from build123d import *

# Parameters (mm, degrees)
SKETCH1_W               = 19.5
SKETCH1_H               = 7
BOSS_EXTRUDE1_DEPTH     = 3
CUT_EXTRUDE1_DEPTH      = 7
CUT_EXTRUDE2_DEPTH      = 21.934421415
CUT_EXTRUDE2_DEPTH_BACK = 21.934421415
SKETCH4_R               = 1.8
CUT_EXTRUDE3_DEPTH      = 0.8


with BuildPart() as part:
    # Sketch1 → Boss-Extrude1 (new body)
    with BuildSketch(Plane(origin=(0, 0, 0), x_dir=(1, 0, 0), z_dir=(0, 1, 0))):
        with Locations((9.75, 3.5)):
            Rectangle(SKETCH1_W, SKETCH1_H)
    extrude(amount=BOSS_EXTRUDE1_DEPTH)

    # Sketch2 → Cut-Extrude1 (cut)
    with BuildSketch(Plane.XY):
        Polygon((0, 0), (0.7, 3), (0, 3), align=None)
        Polygon((19.5, 0), (18.8, 3), (19.5, 3), align=None)
    extrude(amount=-CUT_EXTRUDE1_DEPTH, mode=Mode.SUBTRACT)

    # Sketch3 → Cut-Extrude2 (cut, two sides: drawn at the far end of the back side and taken through both)
    with BuildSketch(Plane(origin=(0, 0, 0), x_dir=(0, 0, -1), z_dir=(1, 0, 0)).offset(-CUT_EXTRUDE2_DEPTH_BACK)):
        Polygon((0, 0), (0.7, 3), (0, 3), align=None)
        Polygon((7, 3), (6.3, 3), (7, 0), align=None)
    extrude(amount=CUT_EXTRUDE2_DEPTH + CUT_EXTRUDE2_DEPTH_BACK, mode=Mode.SUBTRACT)

    # Sketch4 → Cut-Extrude3 (cut)
    with BuildSketch(Plane.XZ):
        with Locations(Location((9.75, -3.5, 0), (0, 0, 270))):
            Circle(SKETCH4_R)
    extrude(amount=-CUT_EXTRUDE3_DEPTH, mode=Mode.SUBTRACT)


solid = part.part
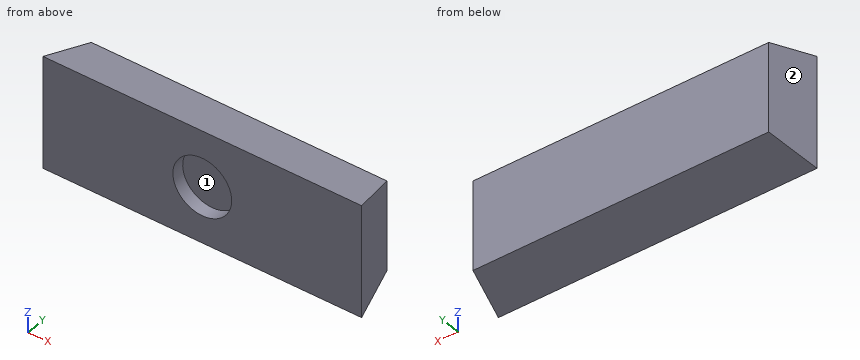
Verification items for the finished model (mm, model axes). Face numbers are marked on the shaded views. Give positions to 0.01 mm unless a question says otherwise; leave off trailing zeros. Order: outer loops, then holes, each group sorted by start corner. A loop starts at its lowest first (then second) coordinate and runs counter-clockwise, first axis right, second up. Notation, with made-up numbers: (89, -29) -> (118, -29) arc R19 ccw to (118, -24) -> close; hole circle Ø2 at (19, 13.25). An arc over 180 degrees is marked (long way). Answer as CSV lines item,"result".
Q1. Scan lines: probe 1 along Y at (x, z) = (9.5, -4.25); probe 2 along X at (y, z) = (0.4, -3.5); probe 3 along Z at (x, y) = (8.5, 0.3). Record each from-to range of solid material in increasing order.
Solutions:
probe 1,"y = 0.8 to 3"
probe 2,"x = 0.09 to 7.95, 11.55 to 19.41"
probe 3,"z = -6.93 to -4.8, -2.2 to -0.07"
Q2. Depth check by flat-ended pin: pin 1 (1.5 mm diameter, centred on y = 1, z = -2.5, fed in from -X). Enter the tip coordinate at first touch or a pass-through.
Solutions:
pin 1,"stops at x = 0.06"
Q3. Sectioned sample at B-B on z = -3.5. Record the cut outline in (x, y), plus the area to 3 significant figures.
Solutions:
outline,"(0, 0) -> (7.95, 0) -> (7.95, 0.8) -> (11.55, 0.8) -> (11.55, 0) -> (19.5, 0) -> (18.8, 3) -> (0.7, 3) -> close"
area,"53.5 mm²"
Q4. Release check for a two-part mould opening along Y. For the marked faces 1 and 2 record: +Y half, -Y half, draft (parallel to the pull), parting line (faces both ways), or undercut.
Solutions:
face 1,"-Y half"
face 2,"+Y half"
Q5. Sectioned sample at D-D on x = 14.5. Record the cut outline in (y, z).
Solutions:
outline,"(0, -7) -> (3, -6.3) -> (3, -0.7) -> (0, 0) -> close"
Q6. Sectioned sample at A-A on x = 9.75. Record the cut outline in (y, z).
Solutions:
outline,"(0, -7) -> (3, -6.3) -> (3, -0.7) -> (0, 0) -> (0, -1.7) -> (0.8, -1.7) -> (0.8, -5.3) -> (0, -5.3) -> close"
Q7. Sectioned sample at C-C on y = 0.2. Record the cut outline in (x, z), plus the area to 3 significant figures.
Solutions:
outline,"(0.05, -6.95) -> (19.45, -6.95) -> (19.45, -0.05) -> (0.05, -0.05) -> close; hole circle Ø3.6 at (9.75, -3.5)"
area,"124 mm²"
